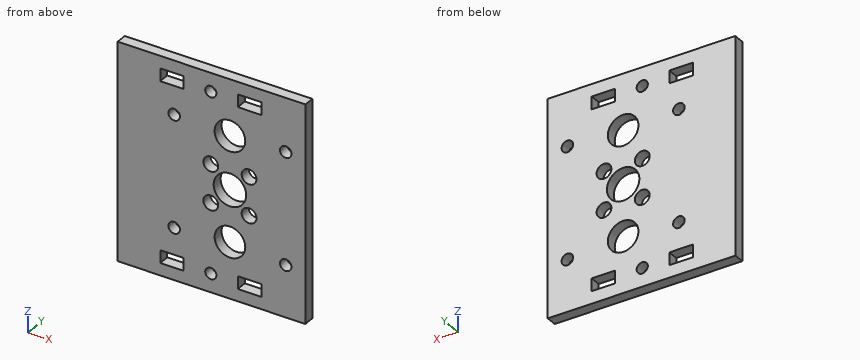
Autodesk Inventor part; units mm, degrees
ref_plane "YZ Plane" through (0, 0, 0) normal (1, 0, 0) x (0, 1, 0)
ref_plane "XZ Plane" through (0, 0, 0) normal (0, 1, 0) x (-1, 0, 0)
ref_plane "XY Plane" through (0, 0, 0) normal (0, 0, 1) x (1, 0, 0)
sketch "Sketch1" plane through (0, 0, 0) normal (0, 1, 0) x (-1, 0, 0)
  line L0 (0, 0) -> (52, 0)
  line L1 (52, 0) -> (52, 60)
  line L2 (52, 60) -> (0, 60)
  line L3 (0, 60) -> (0, 0)
  dimension "d0" = 52
  dimension "d1" = 60
extrude "Extrusion1" add sketch "Sketch1" along normal blind 3
sketch "Sketch2" plane through (0, 3, 0) normal (0, 1, 0) x (1, 0, 0)
  line L0 (-52, 0) -> (-52, -60)
  line L1 (-52, 0) -> (-40.2, 0)
  line L2 (-40.2, 0) -> (-40.2, -3.4)
  line L3 (-40.2, -3.4) -> (-52, -3.4)
  line L4 (-52, -3.4) -> (-52, 0)
  line L5 (-40.2, -3.4) -> (-33.7, -3.4)
  line L6 (-33.7, -3.4) -> (-33.7, -6.9)
  line L7 (-33.7, -6.9) -> (-40.2, -6.9)
  line L8 (-40.2, -6.9) -> (-40.2, -3.4)
  line L9 (-33.7, -3.4) -> (-18.7, -3.4)
  line L10 (-18.7, -3.4) -> (-12.2, -3.4)
  line L11 (-12.2, -3.4) -> (-12.2, -6.9)
  line L12 (-12.2, -6.9) -> (-18.7, -6.9)
  line L13 (-18.7, -6.9) -> (-18.7, -3.4)
  line L14 (-52, -30) -> (0, -30)
  line L15 (0, -60) -> (0, 0)
  line L16 (-40.2, -56.6) -> (-33.7, -56.6)
  line L17 (-33.7, -56.6) -> (-33.7, -53.1)
  line L18 (-33.7, -53.1) -> (-40.2, -53.1)
  line L19 (-40.2, -53.1) -> (-40.2, -56.6)
  line L20 (-18.7, -56.6) -> (-12.2, -56.6)
  line L21 (-12.2, -56.6) -> (-12.2, -53.1)
  line L22 (-12.2, -53.1) -> (-18.7, -53.1)
  line L23 (-18.7, -53.1) -> (-18.7, -56.6)
  dimension "d4" = 11.8
  dimension "d5" = 3.4
  dimension "d6" = 6.5
  dimension "d7" = 3.5
  dimension "d8" = 15
  dimension "d9" = 6.5
  dimension "d10" = 3.5
extrude "Extrusion2" cut sketch "Sketch2" against normal blind 3 contours L10 L11 L12 L13 | L5 L6 L7 L8 | L19 L18 L17 L16 | L23 L22 L21 L20
sketch "Sketch3" plane through (0, 3, 0) normal (0, 1, 0) x (1, 0, 0)
  line L0 (-52, -60) -> (0, -60)
  line L1 (-52, -60) -> (-20.9, -60)
  line L2 (-20.9, -60) -> (-20.9, -44.5)
  line L3 (-20.9, -44.5) -> (-52, -44.5)
  line L4 (-52, -44.5) -> (-52, -60)
  circle A0 centre (-20.9, -44.5) radius 4.25
  line L5 (-52, 0) -> (-52, -60)
  line L6 (-52, -30) -> (0, -30)
  line L7 (0, -60) -> (0, 0)
  circle A1 centre (-20.9, -15.5) radius 4.25
  dimension "d13" = 31.1
  dimension "d14" = 15.5
  dimension "d15" = 8.5
extrude "Extrusion3" cut sketch "Sketch3" against normal blind 3 contours A0 L3 L2 | L2 L3 A0 | A1
sketch "Sketch4" plane through (0, 3, 0) normal (0, 1, 0) x (1, 0, 0)
  circle A0 centre (-20.9, -44.5) radius 4.25
  line L0 (-20.9, -40.25) -> (-20.9, -29.75)
  circle A1 centre (-20.9, -29.75) radius 4.5
  point P0 (0, 0)
  dimension "d18" = 10.5
  dimension "d19" = 9
extrude "Extrusion4" cut sketch "Sketch4" against normal blind 3 contours A1
sketch "Sketch5" plane through (0, 3, 0) normal (0, 1, 0) x (1, 0, 0)
  circle A0 centre (-20.9, -29.75) radius 4.5
  line L0 (-20.9, -29.75) -> (-26.2033, -35.0533)
  line L1 (-20.9, -29.75) -> (-13.4, -29.75) construction
  circle A1 centre (-26.2033, -35.0533) radius 2.05
  point P0 (0, 0)
  dimension "d22" = 7.5
  dimension "d23" = 135
  dimension "d24" = 4.1
extrude "Extrusion5" cut sketch "Sketch5" against normal blind 3 contours A1
pattern_circular "Circular Pattern1" count 4 over 360 about axis through (-20.9, 3, 29.75) along (0, -1, 0) of "Extrusion5"
sketch "Sketch6" plane through (0, 3, 0) normal (0, 1, 0) x (1, 0, 0)
  circle A0 centre (-20.9, -29.75) radius 4.5
  line L0 (-20.9, -29.75) -> (-5.4497, -45.2003)
  line L1 (-20.9, -29.75) -> (0.95, -29.75) construction
  circle A1 centre (-5.4497, -45.2003) radius 1.6
  line L2 (-20.9, -29.75) -> (-5.4497, -14.2997)
  line L3 (-20.9, -29.75) -> (-36.3503, -45.2003)
  line L4 (-20.9, -29.75) -> (-36.3503, -14.2997)
  circle A2 centre (-36.3503, -45.2003) radius 1.6
  circle A3 centre (-36.3503, -14.2997) radius 1.6
  circle A4 centre (-5.4497, -14.2997) radius 1.6
  point P0 (0, 0)
  dimension "d30" = 21.85
  dimension "d31" = 45
  dimension "d32" = 3.2
  dimension "d35" = 21.85
  dimension "d36" = 21.85
  dimension "d37" = 21.85
  dimension "d38" = 3.2
  dimension "d39" = 3.2
  dimension "d40" = 3.2
extrude "Extrusion6" cut sketch "Sketch6" against normal blind 3.2 contours A1 | A2 | A3 | A4
sketch "Sketch7" plane through (0, 3, 0) normal (0, 1, 0) x (1, 0, 0)
  line L0 (-33.7, -6.9) -> (-33.7, -3.4)
  line L1 (-33.7, -5.15) -> (-26.2, -5.15)
  line L2 (-52, 0) -> (-52, -60)
  line L3 (-52, -30) -> (-2, -30)
  circle A0 centre (-26.2, -5.15) radius 1.55
  circle A1 centre (-26.2, -54.85) radius 1.55
  point P0 (0, 0)
  dimension "d41" = 7.5
  dimension "d42" = 50
  dimension "d43" = 3.1
extrude "Extrusion7" cut sketch "Sketch7" against normal blind 3.1
equation "\"d33\" = d39"
equation "\"d44\" = d43"
properties part number "pumpeplade"
Verification items for the finished model (mm, model axes). Round coordinates to 2 decimals unless told otherwise and drop trailing zeros. Order: outer loops, then holes, each group sorted by start corner. A loop starts at its lowest first (then second) coordinate and runs counter-clockwise, first axis right, second up. Notation, with made-up numbers: (-31.75, 17) -> (20.25, 17) arc R32 ccw to (20.25, 56) -> close; hole circle Ø5 at (27.25, -23). An arc over 180 degrees is marked (long way). Put each result on its own line as item: value. Start each with the question number.
(1) Section check C-C (z = 29.75). Enter the section's corners in (x, y).
(2) Section check A-A (z = 54.85). Enter the section's corners in (x, y), then the cut area to 3 significant figures.
(3) Section check D-D (y = 0.5). State how many separate pieces and enclosed holes the cut face has, then the cut area to 3 significant figures.
(4) Depth check by flat-ended pin: pin 1 Ø2.5 at (x, z) = (-26.2, 35.05) entering from -Y. Enter the tip coordinate at first touch or a pass-through.
(5) Section check B-B (x = -20.9). Enter the section's corners in (y, z), then the cut area to 3 significant figures.
(6) Material ranges on line 1 along Z through (x, y) = (-38.5, 0.4); line 2 along Z through (x, y) = (-20.9, 0.8); line 3 along X through (y, z) = (1.35, 54.85), recorded low to high.
Completed:
1. outline: (-52, 0) -> (-25.4, 0) -> (-25.4, 3) -> (-52, 3) -> close; (-16.4, 0) -> (0, 0) -> (0, 3) -> (-16.4, 3) -> close
2. outline: (-52, 0) -> (-40.2, 0) -> (-40.2, 3) -> (-52, 3) -> close; (-33.7, 0) -> (-27.75, 0) -> (-27.75, 3) -> (-33.7, 3) -> close; (-24.65, 0) -> (-18.7, 0) -> (-18.7, 3) -> (-24.65, 3) -> close; (-12.2, 0) -> (0, 0) -> (0, 3) -> (-12.2, 3) -> close
2. area: 108 mm2
3. separate pieces: 1
3. enclosed holes: 17
3. area: 2,750 mm2
4. pin 1: passes through
5. outline: (0, 0) -> (3, 0) -> (3, 11.25) -> (0, 11.25) -> close; (0, 19.75) -> (3, 19.75) -> (3, 25.25) -> (0, 25.25) -> close; (0, 34.25) -> (3, 34.25) -> (3, 40.25) -> (0, 40.25) -> close; (0, 48.75) -> (3, 48.75) -> (3, 60) -> (0, 60) -> close
5. area: 102 mm2
6. line 1: z = 0 to 3.4, 6.9 to 53.1, 56.6 to 60
6. line 2: z = 0 to 11.25, 19.75 to 25.25, 34.25 to 40.25, 48.75 to 60
6. line 3: x = -52 to -40.2, -33.7 to -27.75, -24.65 to -18.7, -12.2 to 0
